from build123d import *

# Parameters (mm, degrees)
SKETCH1_R           = 13
BOSS_EXTRUDE1_DEPTH = 1
SKETCH16_R          = 13
BOSS_EXTRUDE3_DEPTH = 1
SKETCH19_R          = 1
BOSS_EXTRUDE4_DEPTH = 29.8
SKETCH18_W          = 22
SKETCH18_H          = 22
CUT_EXTRUDE6_DEPTH  = 3.7
SKETCH21_W          = 22
SKETCH21_H          = 22
CUT_EXTRUDE7_DEPTH  = 3.7
SKETCH22_R          = 11
CUT_EXTRUDE8_DEPTH  = 3.7
SKETCH23_R          = 11
CUT_EXTRUDE9_DEPTH  = 3.7
SKETCH24_R          = 19.921792127
CUT_EXTRUDE10_DEPTH = 1
SKETCH25_R          = 36.182885583
CUT_EXTRUDE11_DEPTH = 1
BOSS_EXTRUDE5_START = 2
BOSS_EXTRUDE5_DEPTH = 2
SKETCH27_R          = 1
BOSS_EXTRUDE6_DEPTH = 2
SKETCH28_R          = 9.676669919
CUT_EXTRUDE12_DEPTH = 17.4


with BuildPart() as part:
    # Sketch1 → Boss-Extrude1 (new body)
    with BuildSketch(Plane(origin=(0, 0, 0), x_dir=(1, 0, 0), z_dir=(0, 1, 0))):
        with Locations(Location((0, 0, 0), (0, 0, 270))):
            Circle(SKETCH1_R)
    extrude(amount=BOSS_EXTRUDE1_DEPTH)



with BuildPart() as body_2:
    # Sketch16 → Boss-Extrude3 (new body)
    with BuildSketch(Plane(origin=(0, 30.8, 0), x_dir=(1, 0, 0), z_dir=(0, 1, 0))):
        with Locations(Location((0, 0, 0), (0, 0, 270))):
            Circle(SKETCH16_R)
    extrude(amount=BOSS_EXTRUDE3_DEPTH)


with BuildPart() as part_1:
    add(part.part)

    add(body_2.part)  # Boss-Extrude4 merges body 2
    # Sketch19 → Boss-Extrude4 (add)
    with BuildSketch(Plane(origin=(0, 1, 0), x_dir=(1, 0, 0), z_dir=(0, 1, 0))):
        with Locations(Location((0, 11, 0), (0, 0, 270))):
            Circle(SKETCH19_R)
    extrude(amount=BOSS_EXTRUDE4_DEPTH)

    # Sketch18 → Cut-Extrude6 (cut)
    with BuildSketch(Plane(origin=(0, 4.7, 0), x_dir=(1, 0, 0), z_dir=(0, 1, 0))):
        Rectangle(SKETCH18_W, SKETCH18_H)
    extrude(amount=-CUT_EXTRUDE6_DEPTH, mode=Mode.SUBTRACT)

    # Sketch21 → Cut-Extrude7 (cut)
    with BuildSketch(Plane(origin=(0, 13.4, 0), x_dir=(1, 0, 0), z_dir=(0, 1, 0))):
        Rectangle(SKETCH21_W, SKETCH21_H)
    extrude(amount=-CUT_EXTRUDE7_DEPTH, mode=Mode.SUBTRACT)

    # Sketch22 → Cut-Extrude8 (cut)
    with BuildSketch(Plane(origin=(0, 22.1, 0), x_dir=(1, 0, 0), z_dir=(0, 1, 0))):
        Circle(SKETCH22_R)
    extrude(amount=-CUT_EXTRUDE8_DEPTH, mode=Mode.SUBTRACT)

    # Sketch23 → Cut-Extrude9 (cut)
    with BuildSketch(Plane(origin=(0, 30.8, 0), x_dir=(1, 0, 0), z_dir=(0, 1, 0))):
        Circle(SKETCH23_R)
    extrude(amount=-CUT_EXTRUDE9_DEPTH, mode=Mode.SUBTRACT)

    # Sketch24 → Cut-Extrude10 (cut)
    with BuildSketch(Plane(origin=(0, 31.8, 0), x_dir=(1, 0, 0), z_dir=(0, 1, 0))):
        Circle(SKETCH24_R)
    extrude(amount=-CUT_EXTRUDE10_DEPTH, mode=Mode.SUBTRACT)

    # Sketch25 → Cut-Extrude11 (cut)
    with BuildSketch(Plane(origin=(0, 1, 0), x_dir=(1, 0, 0), z_dir=(0, 1, 0))):
        Circle(SKETCH25_R)
    extrude(amount=-CUT_EXTRUDE11_DEPTH, mode=Mode.SUBTRACT)

    # Sketch26 → Boss-Extrude5 (add)
    with BuildSketch(Plane(origin=(0, 30.8, 0), x_dir=(1, 0, 0), z_dir=(0, 1, 0)).offset(BOSS_EXTRUDE5_START)):
        with BuildLine():
            ThreePointArc((-0.998966408, 10.954545455), (0, 11), (0.998966408, 10.954545455))
            ThreePointArc((0.998966408, 10.954545455), (0, 12), (-0.998966408, 10.954545455))
        make_face()
        with BuildLine():
            ThreePointArc((0.998966408, 10.954545455), (0.999741569, 10.977266852), (1, 11))
            ThreePointArc((1, 11), (-0.022733148, 11.999741569), (-0.998966408, 10.954545455))
            ThreePointArc((-0.998966408, 10.954545455), (0, 11), (0.998966408, 10.954545455))
        make_face()
        with BuildLine():
            ThreePointArc((0.998966408, 10.954545455), (0, 11), (-0.998966408, 10.954545455))
            ThreePointArc((-0.998966408, 10.954545455), (0, 10), (0.998966408, 10.954545455))
        make_face()
    extrude(amount=-BOSS_EXTRUDE5_DEPTH)

    # Sketch27 → Boss-Extrude6 (add)
    with BuildSketch(Plane.XZ.offset(-1)):
        with Locations(Location((0, -11, 0), (0, 0, 270))):
            Circle(SKETCH27_R)
    extrude(amount=BOSS_EXTRUDE6_DEPTH)

    # Sketch28 → Cut-Extrude12 (cut)
    with BuildSketch(Plane(origin=(0, 32.8, 0), x_dir=(1, 0, 0), z_dir=(0, 1, 0))):
        with Locations((0, 11)):
            Circle(SKETCH28_R)
    extrude(amount=-CUT_EXTRUDE12_DEPTH, mode=Mode.SUBTRACT)


solid = part_1.part
Design review of the part built by this model. Coordinates are the model's own, in mm. Coordinates: 2 decimals unless noted, no trailing zeros. Order: outer loops, then holes, each group sorted by start corner. A loop starts at its lowest first (then second) coordinate and runs counter-clockwise, first axis right, second up. Notation, with made-up numbers: (83.5, -32.5) -> (89.5, -32.5) arc R24 ccw to (89.5, -12.5) -> close; hole circle Ø8 at (80.25, -37). An arc over 180 degrees is marked (long way). One line per item, written item: value.
1) Clearance check with a flat-ended pin moving along its axis: P1, Ø0.6, axis at x = 0, y = 10.5, coming from the +Z side. State where the tip first meets the part, or that it passes through.
Output values:
P1: stops at z = -11
2) We need section C-C, the plane y = 5.25. Give the boundary of the cut face in (x, z).
Output values:
outline: circle Ø2 at (0, -11)
3) We need section B-B, the plane z = -10.3. Give the boundary of the cut face in (x, y).
Output values:
outline: (-0.71, -1) -> (0.71, -1) -> (0.71, 1) -> (-0.71, 1) -> close; (-0.71, 4.7) -> (0.71, 4.7) -> (0.71, 9.7) -> (-0.71, 9.7) -> close; (-0.71, 13.4) -> (0.71, 13.4) -> (0.71, 15.4) -> (-0.71, 15.4) -> close
4) Draft analysis for pull direction Y (two halves, no side actions). For faces 1 (the face through (0, 3, -11)), 2 (the face through (0, 15.4, -11)), 3 (the face through (0, 12, -11)), 4 (the face through (0, -1, -11)), state which applies: +Y half, -Y half, draft (parallel to the pull), parting line (faces both ways), or undercut.
Output values:
face 1: undercut
face 2: +Y half
face 3: undercut
face 4: -Y half
5) We need section A-A, the plane x = -0.6. Give the boundary of the cut face in (y, z), then the cut area to 3 significant figures.
Output values:
outline: (-1, -11.8) -> (15.4, -11.8) -> (15.4, -10.2) -> (13.4, -10.2) -> (13.4, -11) -> (9.7, -11) -> (9.7, -10.2) -> (4.7, -10.2) -> (4.7, -11) -> (1, -11) -> (1, -10.2) -> (-1, -10.2) -> close
area: 20.3 mm2
6) We need section D-D, the plane x = 0. Give the boundary of the cut face in (y, z), then the cut area to 3 significant figures.
Output values:
outline: (-1, -12) -> (15.4, -12) -> (15.4, -10) -> (13.4, -10) -> (13.4, -11) -> (9.7, -11) -> (9.7, -10) -> (4.7, -10) -> (4.7, -11) -> (1, -11) -> (1, -10) -> (-1, -10) -> close
area: 25.4 mm2
7) To check wall thickness, follow probe 1 along Y at (x, z) = (-0.55, -10.7); probe 2 along Z at (x, y) = (0, 10.25); probe 3 along Z at (x, y) = (0.7, 10.5). State the ranges of each line that lie inside material, in increasing order. Write a range as [from, to].
Output values:
probe 1: y = [-1, 1], [4.7, 9.7], [13.4, 15.4]
probe 2: z = [-12, -11]
probe 3: z = [-11.71, -11]
